The figure shows three views and two pictorial views of one solid part (mm, origin at its lowest corner). Answer the questions. Coordinates: 2 decimals unless noted, no trailing zeros. Loops run counter-clockwise (first coordinate to the right, second up) from the corner with the lowest first, then second, coordinate; pieces in that order, holes last. Notation, with made-up numbers: (34, 79.25) - (49, 79.25) arc R25 cw to (49, 109.25) - close; hole circle Ø5 at (7.25, 53.25). An arc over 180 degrees is marked (long way). One line per question, with ' | ' between items.
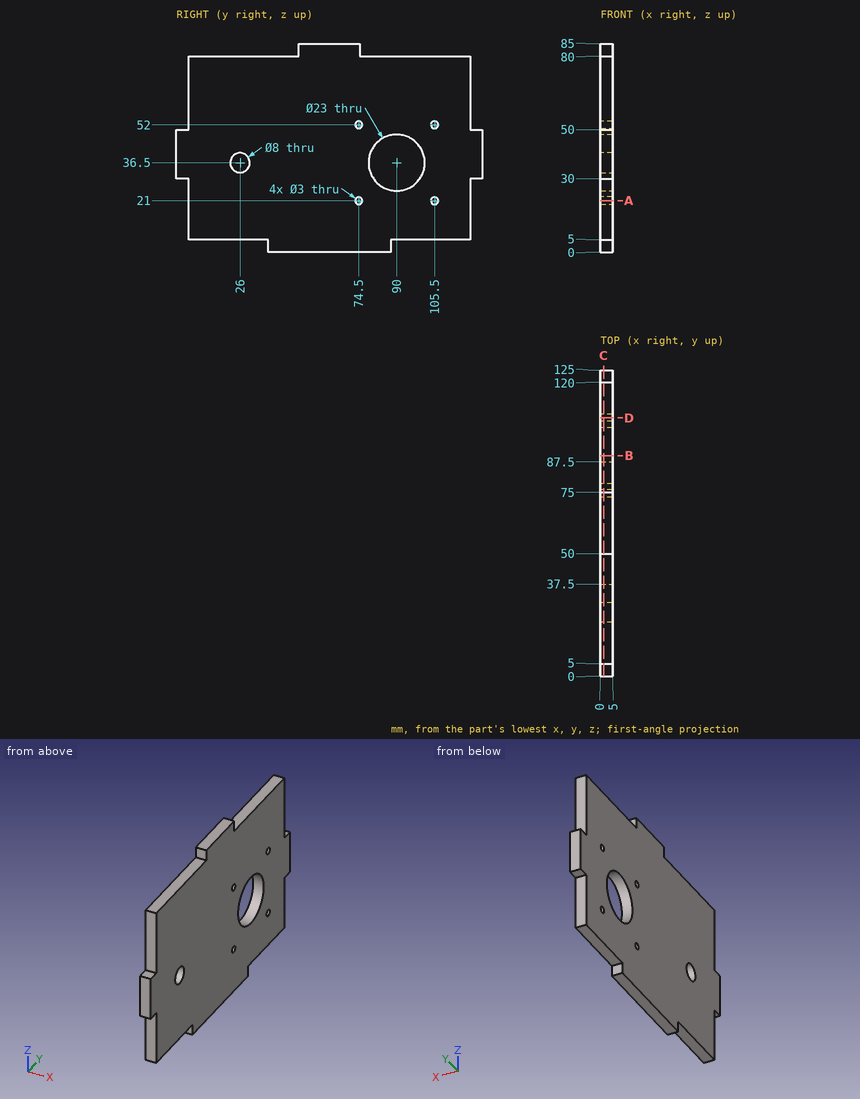
Item 1: Each of these flat-tipped pins is pushed along its axis until it touches: pin 1 Ø2.5 at (x, y) = (2, 89.5) entering from +Z; pin 2 Ø1.5 at (x, z) = (3.5, 21.5) entering from -Y; pin 3 Ø2 at (x, z) = (1, 52.5) entering from +Y. Where does it stop, or does it pass through?
Taken from the geometry:
pin 1: stops at z = 80 | pin 2: stops at y = 5 | pin 3: stops at y = 120
Item 2: Find section D-D, the plane y = 105.5. Write down the section's boundary in (x, z), plus the area to 3 significant figures.
Taken from the geometry:
outline: (0, 5) - (5, 5) - (5, 19.5) - (0, 19.5) - close; (0, 22.5) - (5, 22.5) - (5, 50.5) - (0, 50.5) - close; (0, 53.5) - (5, 53.5) - (5, 80) - (0, 80) - close | area: 345 mm2
Item 3: Find section C-C, the plane x = 1.35. Write down the section's boundary in (y, z), plus the area to 3 significant figures.
Taken from the geometry:
outline: (0, 30) - (5, 30) - (5, 5) - (37.5, 5) - (37.5, 0) - (87.5, 0) - (87.5, 5) - (120, 5) - (120, 30) - (125, 30) - (125, 50) - (120, 50) - (120, 80) - (75, 80) - (75, 85) - (50, 85) - (50, 80) - (5, 80) - (5, 50) - (0, 50) - close; hole circle Ø8 at (26, 36.5); hole circle Ø3 at (74.5, 21); hole circle Ø3 at (74.5, 52); hole circle Ø23 at (90, 36.5); hole circle Ø3 at (105.5, 21); hole circle Ø3 at (105.5, 52) | area: 8,710 mm2
Item 4: Find section A-A, the plane z = 21. Write down the section's boundary in (x, y), plus the area to 3 significant figures.
Taken from the geometry:
outline: (0, 5) - (5, 5) - (5, 73) - (0, 73) - close; (0, 76) - (5, 76) - (5, 104) - (0, 104) - close; (0, 107) - (5, 107) - (5, 120) - (0, 120) - close | area: 545 mm2
Item 5: Find the intervals of material crossed by line 1 (Y direction, x = 1.55, z = 36.5); line 2 (Z direction, x = 3.3, y = 74.5); line 3 (Y direction, x = 2.35, z = 21), in increasing order. Write a range as [from, to].
Taken from the geometry:
line 1: y = [0, 22], [30, 78.5], [101.5, 125] | line 2: z = [0, 19.5], [22.5, 50.5], [53.5, 85] | line 3: y = [5, 73], [76, 104], [107, 120]
Item 6: Find section B-B, the plane y = 90. Write down the section's boundary in (x, z), plus the area to 3 significant figures.
Taken from the geometry:
outline: (0, 5) - (5, 5) - (5, 25) - (0, 25) - close; (0, 48) - (5, 48) - (5, 80) - (0, 80) - close | area: 260 mm2
